from build123d import *

# Parameters (mm, degrees)
SKETCH1_R                = 5
BOSS_EXTRUDE1_DEPTH      = 25
SKETCH2_R                = 8
BOSS_EXTRUDE2_DEPTH      = 5
CHAMFER2_SIZE            = 2.5
SKETCH3_R                = 2
CUT_EXTRUDE1_DEPTH       = 10
SKETCH6_W                = 14.643635598
SKETCH6_H                = 6.4
CUT_EXTRUDE2_DEPTH       = 3
CHAMFER4_SIZE            = 1
CHAMFER2_OF_MIRROR4_SIZE = 2.5
CHAMFER4_OF_MIRROR4_SIZE = 1


with BuildPart() as part:
    # Sketch1 → Boss-Extrude1 (new, symmetric)
    with BuildSketch(Plane(origin=(0, 0, 0), x_dir=(1, 0, 0), z_dir=(0, 1, 0))):
        with Locations(Location((0, 0, 0), (0, 0, 270))):
            Circle(SKETCH1_R)
    extrude(amount=BOSS_EXTRUDE1_DEPTH, both=True)

    # Sketch2 → Boss-Extrude2 (add)
    with BuildSketch(Plane(origin=(0, 25, 0), x_dir=(1, 0, 0), z_dir=(0, 1, 0))):
        with Locations(Location((0, 0, 0), (0, 0, 270))):
            Circle(SKETCH2_R)
    boss_extrude2 = extrude(amount=BOSS_EXTRUDE2_DEPTH)

    # Chamfer2
    chamfer2_edges = [part.edges().sort_by_distance(p)[0] for p in [
        (0, 25, -8),
    ]]
    chamfer(chamfer2_edges, length=CHAMFER2_SIZE)

    # Sketch3 → Cut-Extrude1 (cut)
    with BuildSketch(Plane(origin=(0, 30, 0), x_dir=(1, 0, 0), z_dir=(0, 1, 0))):
        with Locations(Location((0, 0, 0), (0, 0, 270))):
            Circle(SKETCH3_R)
    cut_extrude1 = extrude(amount=-CUT_EXTRUDE1_DEPTH, mode=Mode.SUBTRACT)

    # Sketch6 → Cut-Extrude2 (cut)
    with BuildSketch(Plane(origin=(0, 25, 0), x_dir=(-1, 0, 0), z_dir=(0, -1, 0))):
        with Locations((-3.821817799, 0)):
            Rectangle(SKETCH6_W, SKETCH6_H)
    cut_extrude2 = extrude(amount=CUT_EXTRUDE2_DEPTH, mode=Mode.SUBTRACT)

    # Chamfer4
    chamfer4_edges = [part.edges().sort_by_distance(p)[0] for p in [
        (-3.5, 23.5, -3.2),
        (-3.5, 23.5, 3.2),
    ]]
    chamfer(chamfer4_edges, length=CHAMFER4_SIZE)

    # Mirror4: Boss-Extrude2, Cut-Extrude1, Cut-Extrude2 across plane
    add(boss_extrude2.mirror(Plane(origin=(0, 0, 0), x_dir=(0, 0, 1), z_dir=(0, -1, 0))))
    add(cut_extrude1.mirror(Plane(origin=(0, 0, 0), x_dir=(0, 0, 1), z_dir=(0, -1, 0))), mode=Mode.SUBTRACT)
    add(cut_extrude2.mirror(Plane(origin=(0, 0, 0), x_dir=(0, 0, 1), z_dir=(0, -1, 0))), mode=Mode.SUBTRACT)

    # Chamfer2 of Mirror4
    chamfer2_of_mirror4_edges = [part.edges().sort_by_distance(p)[0] for p in [
        (0, -25, -8),
    ]]
    chamfer(chamfer2_of_mirror4_edges, length=CHAMFER2_OF_MIRROR4_SIZE)

    # Chamfer4 of Mirror4
    chamfer4_of_mirror4_edges = [part.edges().sort_by_distance(p)[0] for p in [
        (-3.5, -23.5, -3.2),
        (-3.5, -23.5, 3.2),
    ]]
    chamfer(chamfer4_of_mirror4_edges, length=CHAMFER4_OF_MIRROR4_SIZE)


solid = part.part
The listing builds one solid part. Answer for the finished solid, in the listing's coordinates (mm). A direction names the side the tool comes from. Coordinates: 2 decimals unless noted, no trailing zeros. Loops run counter-clockwise (first coordinate to the right, second up) from the corner with the lowest first, then second, coordinate; pieces in that order, holes last. Notation, with made-up numbers: (43.5, -1.5) -> (85.5, -1.5) arc R20 cw to (85.5, 17.5) -> close; hole circle Ø7 at (31.25, -11.5). An arc over 180 degrees is marked (long way). Write item = value, one per line. Start each with the question number.
1) A cutting plane is placed at B-B (y = -23). Give the vertices of the cut face in (x, z).
2) A cutting plane is placed at C-C (y = 10). Give the vertices of the cut face in (x, z), then the cut area to 3 significant figures.
3) The mould has two halves that part along Y. Classify faces 6 (the face through (-2, -28, 0)), 7 (the face through (-1.69, -25.12, 5.36)), 8 (the face through (1, 24, 3.2)), 9 (the face through (0, 20, 0)): released by +Y, released by -Y, zero draft, split by the parting line, or undercut.
4) Given pin 1 Ø8 at (x, y) = (4, -22) entering from +Z; pin 2 Ø0.9 at (x, y) = (0.5, -23.5) entering from +Z; pin 3 Ø0.9 at (y, z) = (23.5, 0.5) entering from +X, each flat-ended and moving along its own axis, determine where each tip first touches the part or whether it passes through.
5) Straight lines are drawn through the part: line 1 (Y direction, x = -2, z = -0.5); line 2 (Y direction, x = 5.25, z = -1); line 3 (X direction, y = 28.7, z = 0). For each, find the intervals that lie inside material, in ascending order. Write a range as from..to.
6) A tool of negligible diameter and unlimited length cuts with its end or side. For faces 1 (the face through (-2, 28, 0)), 2 (the face through (-2, -30, 2)), 3 (the face through (-4.88, 0.35, -1.08)), 4 (the face through (2, -22, -1)), 5 (the face through (-2, -21, 0)), from which of +Z, -Z, +X, -X, +Y, -Y can it reach the whole face along a straight path? Write none if from no direction.
7) A cutting plane is placed at A-A (z = 0). Count the separate pieces of the cut face and the enclosed holes in it, then the cut area to 4 significant figures.
Responses:
q1.outline = (-3.5, -2.2) -> (-3.5, 2.2) -> (-2.5, 3.2) -> (3.84, 3.2) arc R5 ccw (long way) to (3.84, -3.2) -> (-2.5, -3.2) -> close
q2.outline = circle Ø10 at (0, 0)
q2.area = 78.5 mm²
q3.face_6 = zero draft
q3.face_7 = undercut
q3.face_8 = undercut
q3.face_9 = released by +Y
q4.pin_1 = 5.68
q4.pin_2 = 5
q4.pin_3 = -3.5
q5.line_1 = -30..-25, -22..22, 25..30
q5.line_2 = -30..-25, 25..30
q5.line_3 = -8..-2, 2..8
q6.face_1 = +Y
q6.face_2 = +Z, -Z, +X, -X, -Y
q6.face_3 = none
q6.face_4 = +X
q6.face_5 = -Y
q7.separate_pieces = 3
q7.enclosed_holes = 0
q7.area = 540.5 mm²
